from build123d import *

# Parameters (mm, degrees)
REVOLVE1_ANGLE = 180


with BuildPart() as part:
    # Sketch1 → Revolve1 (revolve)
    with BuildSketch(Plane(origin=(0, 0, 0), x_dir=(1, 0, 0), z_dir=(0, 1, 0))):
        with BuildLine():
            Line((-2.426089026, 0.9), (-1.253621619, 1.331536072))
            ThreePointArc((-1.253621619, 1.331536072), (-1.202626886, 1.345347949), (-1.15, 1.35))
            Line((-1.15, 1.35), (12.217609628, 1.35))
            ThreePointArc((12.217609628, 1.35), (12.359030984, 1.291421356), (12.417609628, 1.15))
            Line((12.417609628, 1.15), (11.317609628, 1.15))
            Line((11.317609628, 1.15), (11.317609628, 0.9))
            Line((11.317609628, 0.9), (3.617609628, 0.9))
            Line((3.617609628, 0.9), (3.617609628, 0.3))
            Line((3.617609628, 0.3), (2.917609628, 0.3))
            Line((2.917609628, 0.3), (2.917609628, 0.9))
            Line((2.917609628, 0.9), (-0.754449261, 0.9))
            Line((-0.754449261, 0.9), (-1.15, 0.56))
            Line((-1.15, 0.56), (-2.082390372, 0.56))
            Line((-2.082390372, 0.56), (-2.082390372, 0.3))
            Line((-2.082390372, 0.3), (-2.622467407, 0.3))
            Line((-2.622467407, 0.3), (-2.622467407, 0.618463928))
            ThreePointArc((-2.622467407, 0.618463928), (-2.568522772, 0.790093637), (-2.426089026, 0.9))
        make_face()
    revolve(axis=Axis((-3.185032955, 0, -0.1), (-1, 0, 0)), revolution_arc=REVOLVE1_ANGLE)


solid = part.part
Source: CAD feature listing. Evaluate the final solid. Frame: model axes, mm. A direction names the side the tool comes from. Coordinates: 2 decimals unless noted, no trailing zeros. Loops run counter-clockwise (first coordinate to the right, second up) from the corner with the lowest first, then second, coordinate; pieces in that order, holes last. Notation, with made-up numbers: M 63,-31 L 98,-31 A28 cw 98,-10 Z; hole C 1,54 d5. An arc over 180 degrees is marked long. Answer in a Markdown table with one row per item.
Q1. Ray query, probe 1 along Z at (x, y) = (8.5, -0.05); probe 2 along X at (y, z) = (-0.65, -0.5); probe 3 along X at (y, z) = (-0.15, -0.5). Return the intervals inside material, ascending. Write a range as from..to.
Answers below:
| item | result |
|---|---|
| probe 1 | z = -1.35..-0.9, 0.7..1.15 |
| probe 2 | x = -2.5..-0.8, 2.92..3.62 |
| probe 3 | x = -2.62..-2.08, 2.92..3.62 |
Q2. First-contact query: pin 1 (0.6 mm diameter, centred on y = 0, z = 0, fed in from -X). Flat tip, straight axial feed; report the tip coordinate or a pass-through.
Answers below:
| item | result |
|---|---|
| pin 1 | stops at x = -2.62 |
Q3. Section A-A on z = -0.1. Return the cut outline in (x, y), plus the area to 3 significant figures.
Answers below:
| item | result |
|---|---|
| outline | M -2.62,-0.52 A0.3 ccw -2.43,-0.8 L -1.25,-1.23 A0.3 ccw -1.15,-1.25 L 12.22,-1.25 A0.2 ccw 12.42,-1.05 L 11.32,-1.05 L 11.32,-0.8 L 3.62,-0.8 L 3.62,-0.2 L 2.92,-0.2 L 2.92,-0.8 L -0.75,-0.8 L -1.15,-0.46 L -2.08,-0.46 L -2.08,-0.2 L -2.62,-0.2 Z |
| area | 7.23 mm^2 |
Q4. Draft query along Z for faces 4 (the cylindrical face through (5.63, -1.25, -0.13)), 5 (the flat face through (5, 0, -1.1)), 6 (the cylindrical face through (1.1, -0.8, -0.1)). Return one class per face: pulls with the +Z half, pulls with the -Z half, needs draft (parallel to the pull), parting line crosses it, or undercut.
Answers below:
| item | result |
|---|---|
| face 4 | parting line crosses it |
| face 5 | needs draft |
| face 6 | undercut |
Q5. Section C-C on x = 3.25. Return the cut outline in (y, z).
Answers below:
| item | result |
|---|---|
| outline | M 0,-1.35 L 0,-0.3 A0.2 cw 0,0.1 L 0,1.15 A1.25 ccw Z |
Q6. Section B-B on x = 7.5. Return the cut outline in (y, z), plus the area to 3 significant figures.
Answers below:
| item | result |
|---|---|
| outline | M 0,-1.35 L 0,-0.9 A0.8 cw 0,0.7 L 0,1.15 A1.25 ccw Z |
| area | 1.45 mm^2 |
Q7. Set-up query: faces 1 (the conical face through (-1.96, -0.97, -0.12)), 2 (the cylindrical face through (11.86, -1.05, -0.12)), 3 (the cylindrical face through (-1.62, -0.46, -0.11)). Return all of +Z, -Z, +X, -X, +Y, -Y with unobstructed straight access to the full face (end or side cutting, diameter ignored); none if empty.
Answers below:
| item | result |
|---|---|
| face 1 | -X, -Y |
| face 2 | +X, +Y |
| face 3 | +Y |
